The listing builds one solid part. Answer for the finished solid, in the listing's coordinates (mm). Give positions to 0.01 mm unless a question says otherwise; leave off trailing zeros. Write each loop counter-clockwise with the first axis right and the second up, starting at its lowest first coordinate (ties: lowest second). Pieces come first, ordered by that corner, then holes. Notation, with made-up numbers: (60, -4.75) -> (90, -4.75) arc R17 cw to (90, 15.25) -> close; hole circle Ø1 at (40.5, 6.5). An arc over 180 degrees is marked (long way). Put each result on its own line as item: value. Start each with the question number.
1) A flat-ended cylindrical pin translates along its axis: pin 1 Ø0.6 at (y, z) = (1, 2.5) entering from +X. Find the tip coordinate at first contact, or state that the pin passes through.
2) Find the intervals of material crossed by line 1 along X through (y, z) = (1.15, 16.25); line 2 along Z through (x, y) = (15.5, 1); line 3 along Z through (x, y) = (-30, 0.2), in increasing order. Write a range as from..to.
3) A cutting plane is placed at A-A (z = 2.5). Write down the section's boundary in (x, y), then the cut area to 3 significant figures.
4) A cutting plane is placed at B-B (y = 1.4). Write down the section's boundary in (x, z), then the cut area to 3 significant figures.
5) A cutting plane is placed at C-C (x = 19.5). Write down the section's boundary in (y, z).
6) A cutting plane is placed at D-D (z = 14). Write down the section's boundary in (x, y).
from build123d import *

# Parameters (mm, degrees)
BOSS_EXTRUDE1_DEPTH = 2
SKETCH2_W           = 40.894938579
SKETCH2_H           = 5
CUT_EXTRUDE1_DEPTH  = 2
SKETCH3_R           = 1.24
CUT_EXTRUDE2_DEPTH  = 2
SKETCH4_R           = 1.5
CUT_EXTRUDE3_DEPTH  = 2


with BuildPart() as part:
    # Sketch1 → Boss-Extrude1 (new body)
    with BuildSketch(Plane(origin=(0, 0, 0), x_dir=(1, 0, 0), z_dir=(0, 1, 0))):
        with BuildLine():
            Line((-37.5, 0), (37.5, 0))
            ThreePointArc((37.5, 0), (43.534594906, -9.492944386), (47.551323816, -20))
            Line((47.551323816, -20), (-47.551323816, -20))
            ThreePointArc((-47.551323816, -20), (-43.172342271, -9.675000313), (-37.5, 0))
        make_face()
    extrude(amount=BOSS_EXTRUDE1_DEPTH)

    # Sketch2 → Cut-Extrude1 (cut)
    with BuildSketch(Plane(origin=(0, 2, 0), x_dir=(1, 0, 0), z_dir=(0, 1, 0))):
        with Locations((-0.05253071, -2.5)):
            Rectangle(SKETCH2_W, SKETCH2_H)
    extrude(amount=-CUT_EXTRUDE1_DEPTH, mode=Mode.SUBTRACT)

    # Sketch3 → Cut-Extrude2 (cut)
    with BuildSketch(Plane(origin=(0, 2, 0), x_dir=(1, 0, 0), z_dir=(0, 1, 0))):
        with Locations(Location((-29.814825978, -2.5, 0), (0, 0, 270))):
            Circle(SKETCH3_R)
        with Locations(Location((26.204190081, -2.5, 0), (0, 0, 270))):
            Circle(SKETCH3_R)
        with Locations(Location((-35.574250481, -2.5, 0), (0, 0, 270))):
            Circle(SKETCH3_R)
        with Locations(Location((30.174605265, -2.5, 0), (0, 0, 270))):
            Circle(SKETCH3_R)
        with Locations(Location((33.86984316, -2.5, 0), (0, 0, 270))):
            Circle(SKETCH3_R)
    extrude(amount=-CUT_EXTRUDE2_DEPTH, mode=Mode.SUBTRACT)

    # Sketch4 → Cut-Extrude3 (cut)
    with BuildSketch(Plane(origin=(0, 2, 0), x_dir=(1, 0, 0), z_dir=(0, 1, 0))):
        with Locations(Location((-25.88031453, -17.219701094, 0), (0, 0, 270))):
            Circle(SKETCH4_R)
        with Locations(Location((29.979925966, -17.219701094, 0), (0, 0, 270))):
            Circle(SKETCH4_R)
    extrude(amount=-CUT_EXTRUDE3_DEPTH, mode=Mode.SUBTRACT)


solid = part.part
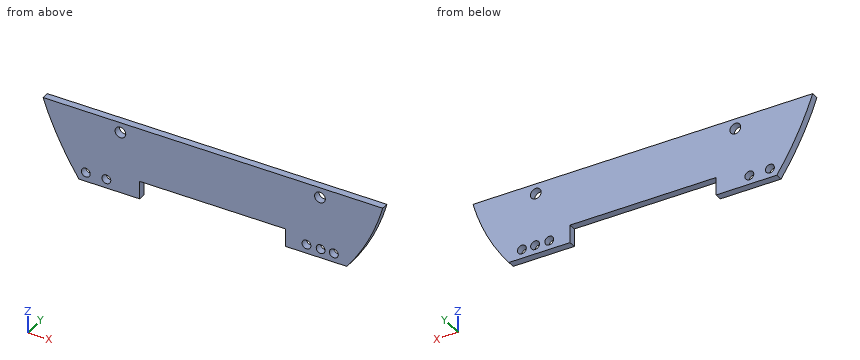
Reply:
1. pin 1: stops at x = 39.57
2. line 1: x = -46.14..-27.02, -24.74..28.84, 31.12..46.39
2. line 2: z = 5..20
2. line 3: z = 0..1.27, 3.73..20
3. outline: (-39.13, 0) -> (-36.81, 0) -> (-36.81, 2) -> (-39.13, 2) -> close; (-34.33, 0) -> (-31.05, 0) -> (-31.05, 2) -> (-34.33, 2) -> close; (-28.57, 0) -> (-20.5, 0) -> (-20.5, 2) -> (-28.57, 2) -> close; (20.39, 0) -> (24.96, 0) -> (24.96, 2) -> (20.39, 2) -> close; (27.44, 0) -> (28.93, 0) -> (28.93, 2) -> (27.44, 2) -> close; (31.41, 0) -> (32.63, 0) -> (32.63, 2) -> (31.41, 2) -> close; (35.11, 0) -> (39.36, 0) -> (39.36, 2) -> (35.11, 2) -> close
3. area: 50.4 mm2
4. outline: (-47.55, 20) arc R86.89 ccw to (-37.5, 0) -> (-20.5, 0) -> (-20.5, 5) -> (20.39, 5) -> (20.39, 0) -> (37.5, 0) arc R56.03 ccw to (47.55, 20) -> close; hole circle Ø2.48 at (-35.57, 2.5); hole circle Ø2.48 at (-29.81, 2.5); hole circle Ø3 at (-25.88, 17.22); hole circle Ø2.48 at (26.2, 2.5); hole circle Ø3 at (29.98, 17.22); hole circle Ø2.48 at (30.17, 2.5); hole circle Ø2.48 at (33.87, 2.5)
4. area: 1,490 mm2
5. outline: (0, 5) -> (2, 5) -> (2, 20) -> (0, 20) -> close
6. outline: (-45.2, 0) -> (45.56, 0) -> (45.56, 2) -> (-45.2, 2) -> close
